```python
from build123d import *

# Parameters (mm, degrees)
F0_W        = 106.7279540002
F0_H        = 43.9982321113
F1_DEPTH    = 71.374
F2_R        = 13.8308303795
F3_DEPTH    = 43.9982321113
F4_T1_DEPTH = 320.8185282784


# Not quite as in the source:
# - a fillet or chamfer that OpenCascade refuses, or shapes differently, is made with other operations: its cross-section is extruded or revolved along the edge and cut away or added


with BuildPart() as f1:
    # F0 (on Top) → F1 (new body)
    with BuildSketch(Plane.XY):
        with Locations((10.7528511435, 12.0171392336)):
            Rectangle(F0_W, F0_H)
    extrude(amount=F1_DEPTH)

    # F2 (on face) → F3 (cut, through all)
    with BuildSketch(Plane.XZ.offset(9.981976822)):
        with Locations((6.3148764893, 38.5243110359)):
            Circle(F2_R)
    extrude(amount=-F3_DEPTH, mode=Mode.SUBTRACT)

    # F4: fillet of radius 50.2832400771 on 1 edges, made by hand

    # F4_s2 → F4_t1 (cut)
    with BuildSketch(Plane.XY.offset(-124.7222641392)):
        with BuildLine():
            ThreePointArc((64.1168281436, 34.0162552893), (47.4873096457, 2.5889655454), (14.2279224879, -9.981976822))
            Line((14.2279224879, -9.981976822), (64.1168281436, -9.981976822))
            Line((64.1168281436, -9.981976822), (64.1168281436, 34.0162552893))
        make_face()
    extrude(amount=F4_T1_DEPTH, mode=Mode.SUBTRACT)


solid = f1.part
```
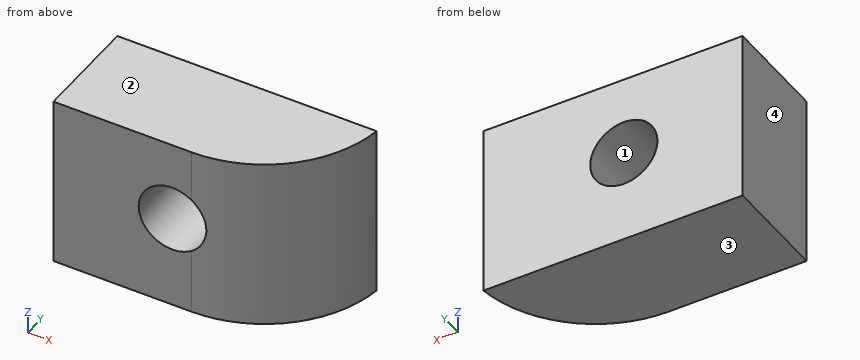
Input: part model. Units: mm. Frame: model coordinates. Face numbers are marked on the shaded views. Round coordinates to 2 decimals unless told otherwise and drop trailing zeros. Loops run counter-clockwise (first coordinate to the right, second up) from the corner with the lowest first, then second, coordinate; pieces in that order, holes last. Notation, with made-up numbers: (71.5, -26) -> (109.5, -26) arc R13 ccw to (109.5, -1) -> close; hole circle Ø3 at (21.25, -32). An arc over 180 degrees is marked (long way). Use one line per item in the form item = value. Start each with the question number.
Item 1: Section query D-D on x = 18. Return the cut outline in (y, z) (3 decimals), then the cut area to 3 significant figures.
Item 2: Section query C-C on y = 9.5. Return the cut outline in (x, z).
Item 3: Section query B-B on x = -3.5. Return the cut outline in (y, z).
Item 4: Contact query for flat-ended pins moving along their axis: pin 1 Ø1 at (y, z) = (6, 24.5) entering from +X; pin 2 Ø10 at (y, z) = (17.5, 38) entering from +X; pin 3 Ø3 at (y, z) = (-4.5, 60.5) entering from +X. Output: stop coordinate, or through.
Item 5: Material intervals for L1, parallel to Z at x = 5, y = 22.5; L2, parallel to Z at x = 10.5, y = 24.5; L3, parallel to Y at x = 43, z = 22, sorted ascending. Write a range as from..to.
Item 6: Mould query, pull axis Z, two halves, no side actions, for the marked faces 1, 2, 3 and 4. Classes: pulls with the +Z half, pulls with the -Z half, needs draft (parallel to the pull), parting line crosses it, or undercut.
Item 7: Section query A-A on z = 45.5. Return the cut outline in (x, y), then the cut area to 3 significant figures.
Ans:
q1.outline = (-9.84, 0) -> (34.016, 0) -> (34.016, 31.125) -> (-9.84, 31.125) -> close; (-9.84, 45.924) -> (34.016, 45.924) -> (34.016, 71.374) -> (-9.84, 71.374) -> close
q1.area = 2,480 mm^2
q2.outline = (-42.61, 0) -> (53.97, 0) -> (53.97, 71.37) -> (-42.61, 71.37) -> close; hole circle Ø27.66 at (6.31, 38.52)
q3.outline = (-9.98, 0) -> (34.02, 0) -> (34.02, 28.78) -> (-9.98, 28.78) -> close; (-9.98, 48.27) -> (34.02, 48.27) -> (34.02, 71.37) -> (-9.98, 71.37) -> close
q4.pin_1 = 51.46
q4.pin_2 = 61.25
q4.pin_3 = 39.79
q5.L1 = 0..24.76, 52.29..71.37
q5.L2 = 0..25.34, 51.71..71.37
q5.L3 = -0.94..34.02
q6.face_1 = undercut
q6.face_2 = pulls with the +Z half
q6.face_3 = pulls with the -Z half
q6.face_4 = needs draft
q7.outline = (-42.61, -9.98) -> (-5.63, -9.98) -> (-5.63, 34.02) -> (-42.61, 34.02) -> close; (18.26, -9.82) arc R50.28 ccw to (64.12, 34.02) -> (18.26, 34.02) -> close
q7.area = 3,120 mm^2
